```python
from build123d import *

# Parameters (mm, degrees)
CYLINDER033_R     = 14
CYLINDER033_DEPTH = 20
BOX_W             = 36
BOX_H             = 16
BOX_DEPTH         = 41
CYLINDER030_R     = 16
CYLINDER030_DEPTH = 28
THICKNESS001_T    = -1


with BuildPart() as cilindro013:
    # Cylinder033 → Cylinder033 (new body)
    with BuildSketch(Plane(origin=(0, 17, 40), x_dir=(1, 0, 0), z_dir=(0, 0, 1))):
        Circle(CYLINDER033_R)
    extrude(amount=CYLINDER033_DEPTH)


with BuildPart() as cubo:
    # Box → Box (new body)
    with BuildSketch(Plane(origin=(-19, 1, 45), x_dir=(1, 0, 0), z_dir=(0, 0, 1))):
        with Locations((18, 8)):
            Rectangle(BOX_W, BOX_H)
    extrude(amount=BOX_DEPTH)


with BuildPart() as cut013016:
    # Cylinder030 → Cylinder030 (new body)
    with BuildSketch(Plane(origin=(0, 17, 45), x_dir=(1, 0, 0), z_dir=(0, 0, 1))):
        Circle(CYLINDER030_R)
    extrude(amount=CYLINDER030_DEPTH)

    # Cut013013: cut Cubo
    add(cubo.part, mode=Mode.SUBTRACT)


with BuildPart() as cut013016_1:
    # Cut013013 placement: moved
    add(cut013016.part.moved(Location((0, 5, 1))))

    # Thickness001
    thickness001_openings = [cut013016_1.faces().sort_by_distance(p)[0] for p in [
        (0, 22, 60),
    ]]
    offset(amount=THICKNESS001_T, openings=thickness001_openings)


with BuildPart() as cut013016_2:
    # Thickness001 placement: moved
    add(cut013016_1.part.moved(Location((0, -5, -2))))

    # Cut013016: cut Cilindro013
    add(cilindro013.part, mode=Mode.SUBTRACT)


solid = cut013016_2.part
```
Model file for the job. Use its own axes, mm. A direction names the side the tool comes from. Round coordinates to 2 decimals unless told otherwise and drop trailing zeros. Order: outer loops, then holes, each group sorted by start corner. A loop starts at its lowest first (then second) coordinate and runs counter-clockwise, first axis right, second up. Notation, with made-up numbers: (-2.75, 77) -> (42.25, 77) arc R15 ccw to (42.25, 97) -> close; hole circle Ø2 at (41.25, -14.5). An arc over 180 degrees is marked (long way). Use one line per item in the form item = value.
Item 1: Tool access for faces 4 (the face through (0, 23, 72)), 5 (the face through (-0.1, 31.2, 45)), 6 (the face through (0.308, 30.997, 44.493)): list every direction of +Z, -Z, +X, -X, +Y, -Y with a clear straight run to the whole face (end or side of a thin tool).
Returned:
face_4 = +Z, +X, -X, +Y, -Y
face_5 = -Y
face_6 = -Z, -Y
Item 2: Cut at A-A, the plane x = 0. Write the cut outline in (y, z), and give its area (3 significant figures).
Returned:
outline = (17, 71) -> (32, 71) -> (32, 45) -> (31, 45) -> (31, 44) -> (33, 44) -> (33, 72) -> (17, 72) -> close
area = 44.0 mm^2
Item 3: Drill centre lines: line 1 (Z direction, x = 12, y = 21.25); line 2 (X direction, y = 18.75, z = 69.5); line 3 (X direction, y = 22.5, z = 67.5). Where is each one in solid material? Low to high.
Returned:
line_1 = 71 to 72
line_2 = -15.9 to -14.9, 14.9 to 15.9
line_3 = -15.02 to -13.96, 13.96 to 15.02
Item 4: Cut at D-D, the plane y = 28.25. Write the cut outline in (x, z), and give its area (3 significant figures).
Returned:
outline = (-11.38, 44) -> (-8.33, 44) -> (-8.33, 45) -> (-9.92, 45) -> (-9.92, 71) -> (9.92, 71) -> (9.92, 45) -> (8.33, 45) -> (8.33, 44) -> (11.38, 44) -> (11.38, 72) -> (-11.38, 72) -> close
area = 105 mm^2
Item 5: Flat gauge pins, fed straight in: pin 1 Ø8 at (x, z) = (-2.5, 68) entering from +Y; pin 2 Ø1 at (y, z) = (21.5, 64.5) entering from +X; pin 3 Ø4 at (x, z) = (5.5, 62) entering from +Y; pin 4 Ø4 at (x, y) = (-0.5, 25) entering from -Z. Where does each tip first touch, or does it go through?
Returned:
pin_1 = 33
pin_2 = 15.49
pin_3 = 32.61
pin_4 = 71
Item 6: Pull direction X, two halves, no side cores. Call faces 1 (the face through (2.3, 31, 44)), 2 (the face through (0, 33, 58)), 3 (the face through (0, 23, 71)): released by +X, released by -X, zero draft, split by the parting line, or undercut.
Returned:
face_1 = zero draft
face_2 = split by the parting line
face_3 = undercut
Item 7: Cut at C-C, the plane z = 67. Write the cut outline in (x, y), and give its area (3 significant figures).
Returned:
outline = (-16, 17) -> (-15, 17) arc R15 cw to (15, 17) -> (16, 17) arc R16 ccw to start
area = 48.7 mm^2
Item 8: Cut at B-B, the plane y = 20. Write the cut outline in (x, z).
Returned:
outline = (-15.72, 44) -> (-13.67, 44) -> (-13.67, 45) -> (-14.7, 45) -> (-14.7, 71) -> (14.7, 71) -> (14.7, 45) -> (13.67, 45) -> (13.67, 44) -> (15.72, 44) -> (15.72, 72) -> (-15.72, 72) -> close
